Input: part model. Units: mm. Frame: model coordinates. A direction names the side the tool comes from. Coordinates: 2 decimals unless noted, no trailing zeros. Order: outer loops, then holes, each group sorted by start corner. A loop starts at its lowest first (then second) coordinate and runs counter-clockwise, first axis right, second up. Notation, with made-up numbers: M -5,-9 L 43,-9 A23 cw 43,4 Z; hole C 49,26.5 d7. An arc over 180 degrees is marked long. Answer in a Markdown table with one row per item.
Autodesk Inventor part; units mm, degrees
ref_plane "YZ Plane" through (0, 0, 0) normal (1, 0, 0) x (0, 1, 0)
ref_plane "XZ Plane" through (0, 0, 0) normal (0, 1, 0) x (-1, 0, 0)
ref_plane "XY Plane" through (0, 0, 0) normal (0, 0, 1) x (1, 0, 0)
sketch "Sketch1" plane through (0, 0, 0) normal (0, 1, 0) x (-1, 0, 0)
  line L0 (0, 0) -> (62.6, 0)
  line L1 (62.6, 0) -> (62.6, -62.6)
  line L2 (62.6, -62.6) -> (0, -62.6)
  line L3 (0, -62.6) -> (0, 0)
  circle A0 centre (31.3, -31.3) radius 2.5
  circle A1 centre (12.25, -12.25) radius 3.1
  circle A2 centre (31.3, -12.25) radius 3.1
  circle A3 centre (50.35, -12.25) radius 3.1
  circle A4 centre (12.25, -50.35) radius 3.1
  circle A5 centre (31.3, -50.35) radius 3.1
  circle A6 centre (50.35, -50.35) radius 3.1
  point P0 (31.3, -62.6)
  dimension "d0" = 62.6
  dimension "d1" = 62.6
  dimension "d2" = 5
  dimension "d3" = 31.3
  dimension "d4" = 31.3
  dimension "d5" = 19.05
  dimension "d6" = 19.05
  dimension "d7" = 6.2
  dimension "d10" = 19.05
  dimension "d13" = 38.1
extrude "Extrusion1" add sketch "Sketch1" along normal blind 11 contours L0 L1 L2 L3 | A0 | A2
sketch "Sketch3" plane through (0, 11, 0) normal (0, 1, 0) x (1, 0, 0)
  circle A0 centre (-31.3, 31.3) radius 2.5
  line L0 (-62.6, 0) -> (0, 0)
  line L1 (0, 0) -> (0, 62.6)
  dimension "d47" = 5
  dimension "d48" = 31.3
  dimension "d49" = 31.3
extrude "Extrusion3" cut sketch "Sketch3" against normal blind 11
sketch "Sketch4" plane through (0, 11, 0) normal (0, 1, 0) x (1, 0, 0)
  circle A0 centre (-31.3, 31.3) radius 2.5
  circle A1 centre (-31.3, 31.3) radius 5.5
  point P0 (0, 0)
  dimension "d52" = 11
sketch "Sketch5" plane through (0, 11, 0) normal (0, 1, 0) x (1, 0, 0)
  circle A0 centre (-12.25, 12.25) radius 3.1
  circle A1 centre (-12.25, 12.25) radius 5.75
  circle A2 centre (-50.35, 12.25) radius 3.1
  circle A3 centre (-50.35, 12.25) radius 5.75
  circle A4 centre (-50.35, 50.35) radius 3.1
  circle A5 centre (-50.35, 50.35) radius 5.75
  circle A6 centre (-31.3, 50.35) radius 3.1
  circle A7 centre (-31.3, 50.35) radius 5.75
  circle A8 centre (-12.25, 50.35) radius 3.1
  circle A9 centre (-12.25, 50.35) radius 5.75
  point P0 (0, 0)
  dimension "d53" = 11.5
  dimension "d54" = 11.5
  dimension "d55" = 11.5
  dimension "d56" = 11.5
  dimension "d57" = 11.5
extrude "Extrusion4" cut sketch "Sketch5" against normal blind 7 contours A0 | A1 | A2 | A3 | A4 | A5 | A7 | A8 | A9
extrude "Extrusion5" cut sketch "Sketch4" against normal blind 8
sketch "Sketch7" plane through (0, 11, 0) normal (0, 1, 0) x (1, 0, 0)
  circle A0 centre (-31.3, 31.3) radius 2.5
  circle A1 centre (-31.3, 31.3) radius 1
  circle A2 centre (-48.7, 31.3) radius 4.05
  circle A3 centre (-13.9, 31.3) radius 4.05
  point P0 (0, 0)
  dimension "d63" = 2
  dimension "d64" = 8.1
  dimension "d65" = 17.4
  dimension "d66" = 8.1
  dimension "d67" = 17.4
extrude "Extrusion6" cut sketch "Sketch7" against normal blind 11 contours A2 | A3
sketch "Sketch8" plane through (0, 11, 0) normal (0, 1, 0) x (1, 0, 0)
  circle A0 centre (-48.7, 31.3) radius 4.05
  circle A1 centre (-48.7, 31.3) radius 6.4
  circle A2 centre (-13.9, 31.3) radius 4.05
  circle A3 centre (-13.9, 31.3) radius 6.4
  point P0 (0, 0)
  point P1 (-44.65, 31.3)
  point P2 (-44.65, 31.3)
  point P3 (-9.85, 31.3)
  point P4 (-9.85, 31.3)
  point P5 (-44.65, 31.3)
  point P6 (-44.65, 31.3)
  dimension "d70" = 12.8
  dimension "d71" = 12.8
extrude "Extrusion7" cut sketch "Sketch8" against normal blind 8.7 contours A0 | A1 | A2 | A3
sketch "Sketch9" plane through (0, 11, 0) normal (0, 1, 0) x (1, 0, 0)
  circle A0 centre (-31.3, 31.3) radius 1
  line L0 (-62.6, 0) -> (0, 0)
  line L1 (0, 0) -> (0, 62.6)
  circle A1 centre (-31.3, 44.8) radius 2.75
  circle A2 centre (-42.9913, 38.05) radius 2.75
  circle A3 centre (-42.9913, 24.55) radius 2.75
  circle A4 centre (-31.3, 17.8) radius 2.75
  circle A5 centre (-19.6087, 24.55) radius 2.75
  circle A6 centre (-19.6087, 38.05) radius 2.75
  dimension "d86" = 2
  dimension "d87" = 31.3
  dimension "d88" = 31.3
  dimension "d89" = 5.5
  dimension "d90" = 13.5
  dimension "d93" = 360
extrude "Extrusion8" cut sketch "Sketch9" against normal blind 11 contours A1 | A2 | A3 | A4 | A5 | A6
chamfer "Chamfer3" distance 3 angle 45 10 edges at (-43.6279, 11, -40.7253) (-41.3597, 11, -35.8363) (-41.3597, 11, -26.7637) (-43.6279, 11, -21.8747) (-34.05, 11, -17.8) (-16.9334, 11, -25.1866) (-21.8223, 11, -22.9184) (-21.8223, 11, -39.6816) (-16.9334, 11, -37.4134) (-31.3, 11, -42.05)
sketch "Sketch10" plane through (0, 0, 0) normal (1, 0, 0) x (0, 0, -1)
  line L0 (62.6, 11) -> (0, 11)
  line L1 (62.6, 11) -> (62.6, 23.3)
  line L2 (62.6, 23.3) -> (51.8, 23.3)
  line L3 (51.8, 23.3) -> (54.2, 11)
  line L4 (54.2, 11) -> (62.6, 11)
  line L5 (0, 11) -> (0, 23.3)
  line L6 (0, 23.3) -> (10.8, 23.3)
  line L7 (10.8, 23.3) -> (8.4, 11)
  point P0 (0, 0)
  dimension "d67" = 17.4
  dimension "d100" = 12.3
  dimension "d101" = 10.8
  dimension "d102" = 8.4
  dimension "d103" = 12.3
  dimension "d104" = 10.8
  dimension "d105" = 8.4
extrude "Extrusion9" add sketch "Sketch10" against normal blind 62.6
sketch "Sketch11" plane through (0, 11, 0) normal (0, 1, 0) x (1, 0, 0)
  circle A0 centre (-50.35, 12.25) radius 5.75
  circle A1 centre (-50.35, 50.35) radius 3.1
  circle A2 centre (-50.35, 50.35) radius 5.75
  arc A3 (-30.3772, 47.3905) -> (-32.2228, 47.3905) centre (-31.3, 50.35) ccw
  circle A4 centre (-31.3, 50.35) radius 5.75
  circle A5 centre (-12.25, 50.35) radius 5.75
  circle A6 centre (-12.25, 12.25) radius 3.1
  circle A7 centre (-12.25, 12.25) radius 5.75
  point P0 (0, 0)
extrude "Extrusion10" cut sketch "Sketch11" along normal blind 62.6 contours A0 | A1 | A2 | A4 | A5 | A6 | A7
equation "\"d4\" = 0.5 * d0"
equation "\"d48\" = 0.5 * d0"
equation "\"d49\" = 0.5 * d1"
equation "\"d66\" = d64"
equation "\"d67\" = d65"
equation "\"d87\" = 0.5 * d1"
equation "\"d88\" = 0.5 * d0"
equation "\"d106\" = d1"
equation "\"d108\" = d1"
properties part number "Tube dovetail bracket"
1) Contact query for flat-ended pins moving along their axis: pin 1 (5 mm diameter, centred on x = -31.3, z = -50.35, fed in from -Y); pin 2 (2 mm diameter, centred on x = -51.5, y = 13.5, fed in from +Z); pin 3 (8 mm diameter, centred on x = -12.25, z = -12.25, fed in from +Y); pin 4 (14 mm diameter, centred on x = -14.5, z = -34, fed in from +Y). Output: stop coordinate, or through.
Resolved:
| item | result |
|---|---|
| pin 1 | passes through |
| pin 2 | stops at z = 0 |
| pin 3 | stops at y = 4 |
| pin 4 | stops at y = 11 |
2) Cut plane C-C, the plane y = 19.75. Output: boundary loops of the cut face in (x, z), and give its area (3 significant figures).
Resolved:
| item | result |
|---|---|
| outline | M -62.6,-62.6 L 0,-62.6 L 0,-52.49 L -6.91,-52.49 A5.75 cw -17.59,-52.49 L -25.96,-52.49 A5.75 cw -36.64,-52.49 L -45.01,-52.49 A5.75 cw -55.69,-52.49 L -62.6,-52.49 Z; M -62.6,-10.11 L -55.69,-10.11 A5.75 cw -45.01,-10.11 L -17.59,-10.11 A5.75 cw -6.91,-10.11 L 0,-10.11 L 0,0 L -62.6,0 Z |
| area | 1,130 mm2 |
3) Mould query, pull axis X, two halves, no side actions, for faces 1 (the face through (-31.408, 3.167, -42.052)), 2 (the face through (-31, 23.3, -5)). Classes: +X half, -X half, draft (parallel to the pull), parting line (faces both ways), or undercut.
Resolved:
| item | result |
|---|---|
| face 1 | undercut |
| face 2 | draft |
4) Material intervals for probe 1 along Z at (x, y) = (-31.3, 6); probe 2 along X at (y, z) = (2.75, -38.05); probe 3 along Z at (x, y) = (-12, 20), sorted ascending.
Resolved:
| item | result |
|---|---|
| probe 1 | z = -62.6 to -56.1, -42.05 to -36.8, -25.8 to -20.55, -15.05 to 0 |
| probe 2 | x = -62.6 to -45.74, -40.24 to -22.36, -16.86 to 0 |
| probe 3 | z = -62.6 to -56.09, -6.51 to 0 |
5) Reachability of faces 3 (the face through (-40.751, 17.236, -52.983)), 4 (the face through (-48, 4, -48)), 5 (the face through (-33.3, 1.5, -29.8)) from +Z, -Z, +X, -X, +Y, -Y: full face, straight path, thin tool, end or side. Return the list, or none.
Resolved:
| item | result |
|---|---|
| face 3 | +X, -X |
| face 4 | +Y |
| face 5 | +Y, -Y |
6) Cut plane B-B, the plane z = -50.35. Output: boundary loops of the cut face in (x, y), and give its area (3 significant figures).
Resolved:
| item | result |
|---|---|
| outline | M -62.6,0 L -53.45,0 L -53.45,4 L -56.1,4 L -56.1,11 L -62.6,11 Z; M -47.25,0 L -34.4,0 L -34.4,4 L -37.05,4 L -37.05,11 L -44.6,11 L -44.6,4 L -47.25,4 Z; M -28.2,0 L -15.35,0 L -15.35,4 L -18,4 L -18,11 L -25.55,11 L -25.55,4 L -28.2,4 Z; M -9.15,0 L 0,0 L 0,11 L -6.5,11 L -6.5,4 L -9.15,4 Z |
| area | 373 mm2 |
7) Cut plane D-D, the plane x = -51. Output: boundary loops of the cut face in (y, z), and give its area (3 significant figures).
Resolved:
| item | result |
|---|---|
| outline | M 0,-62.6 L 23.3,-62.6 L 23.3,-56.06 L 4,-56.06 L 4,-53.38 L 0,-53.38 Z; M 0,-47.32 L 4,-47.32 L 4,-44.64 L 11,-44.64 L 11,-37.27 L 2.3,-37.27 L 2.3,-34.63 L 0,-34.63 Z; M 0,-27.97 L 2.3,-27.97 L 2.3,-25.33 L 11,-25.33 L 11,-17.96 L 4,-17.96 L 4,-15.28 L 0,-15.28 Z; M 0,-9.22 L 4,-9.22 L 4,-6.54 L 23.3,-6.54 L 23.3,0 L 0,0 Z |
| area | 522 mm2 |
8) Cut plane A-A, the plane x = -31.3. Output: boundary loops of the cut face in (y, z).
Resolved:
| item | result |
|---|---|
| outline | M 0,-62.6 L 23.3,-62.6 L 23.3,-56.1 L 4,-56.1 L 4,-53.45 L 0,-53.45 Z; M 0,-42.05 L 8,-42.05 L 11,-39.05 L 11,-36.8 L 3,-36.8 L 3,-33.8 L 0,-33.8 Z; M 0,-28.8 L 3,-28.8 L 3,-25.8 L 11,-25.8 L 11,-23.55 L 8,-20.55 L 0,-20.55 Z; M 0,-15.05 L 8,-15.05 L 11,-12.05 L 11,-8.4 L 23.3,-10.8 L 23.3,0 L 0,0 Z |
